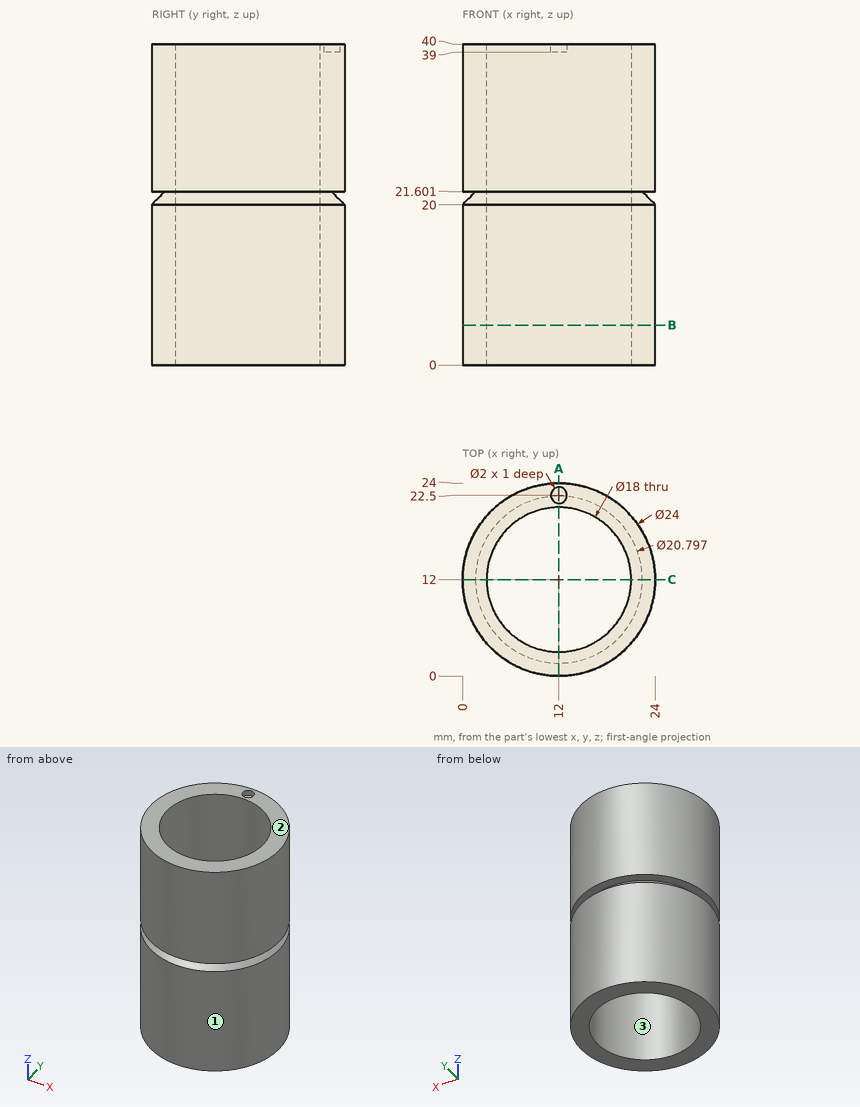
Answer from the drawing. Dimensions are ordinates in mm from the lowest x, y and z of the part. Round coordinates to 2 decimals unless told otherwise and drop trailing zeros. Write each loop counter-clockwise with the first axis right and the second up, starting at its lowest first coordinate (ties: lowest second). Pieces come first, ordered by that corner, then holes. Notation, with made-up numbers: M 70.25,-5.5 L 119.25,-5.5 A25 cw 119.25,30.5 Z; hole C 61,37.5 d1. An arc over 180 degrees is marked long. One line per item, written item: value.
Q1. Straight lines are drawn through the part: line 1 (Y direction, x = 12, z = 39.2); line 2 (Y direction, x = 12, z = 9); line 3 (Z direction, x = 21.5, y = 5.25) (1 decimal). For each, find the intervals that lie inside material, in ascending order. Write a range as [from, to].
Data:
line 1: [0, 3], [21, 21.5], [23.5, 24]
line 2: [0, 3], [21, 24]
line 3: [0, 20.3], [21.6, 40]
Q2. Find section B-B on z = 5. Write down the section's boundary in (x, y), plus the area to 3 significant figures.
Data:
outline: C 12,12 d24; hole C 12,12 d18
area: 198 mm2
Q3. Find section A-A on x = 12. Write down the section's boundary in (y, z).
Data:
outline: M 0,0 L 3,0 L 3,40 L 0,40 L 0,21.6 L 1.6,21.6 L 0,20 Z; M 21,0 L 24,0 L 24,20 L 22.4,21.6 L 24,21.6 L 24,40 L 23.5,40 L 23.5,39 L 21.5,39 L 21.5,40 L 21,40 Z
Q4. For a pull along Y with two mould halves and no side action, classify the marked faces 1, 2 and 3 as +Y half, -Y half, draft (parallel to the pull), parting line (faces both ways), or undercut.
Data:
face 1: parting line
face 2: draft
face 3: undercut
Q5. Flat-ended cylindrical pins translate along their axes: pin 1 Ø1 at (x, y) = (11.5, 22) entering from +Z; pin 2 Ø6 at (y, z) = (16, 33.5) entering from -X; pin 3 Ø5 at (y, z) = (7.5, 33.5) entering from +X; pin 4 Ø8 at (x, z) = (7.5, 27.5) entering from -Y. Find the tip coordinate at first contact, or state that the pin passes through.
Data:
pin 1: z = 40
pin 2: x = 0.04
pin 3: x = 23.83
pin 4: y = 0.01
Q6. Find section C-C on y = 12. Write down the section's boundary in (x, z).
Data:
outline: M 0,0 L 3,0 L 3,40 L 0,40 L 0,21.6 L 1.6,21.6 L 0,20 Z; M 21,0 L 24,0 L 24,20 L 22.4,21.6 L 24,21.6 L 24,40 L 21,40 Z
